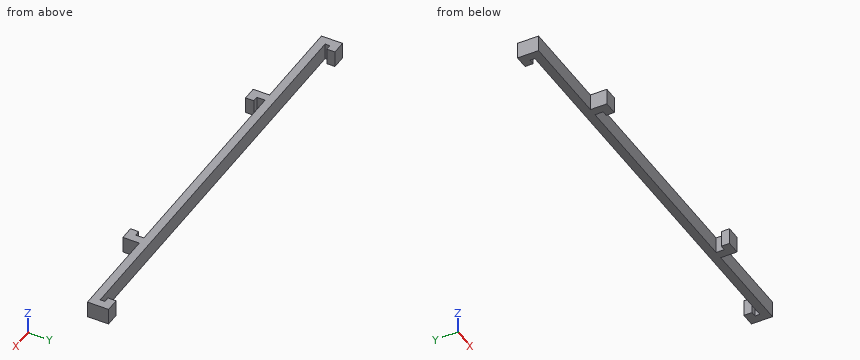
from build123d import *

# Parameters (mm, degrees)
F1_DEPTH = 6


with BuildPart() as f1:
    # F0 (on Top) → F1 (new body)
    with BuildSketch(Plane.XY):
        Polygon((-72.304564, 6.418628), (-72.304564, 9.418628), (-77.304564, 9.418628), (-77.304564, 1.718628), (-43.054564, 1.718628), (-43.054564, -4.281372), (-38.054564, -4.281372), (-38.054564, -1.281372), (-40.054564, -1.281372), (-40.054564, 1.718628), (39.945436, 1.718628), (39.945436, -1.281372), (37.945436, -1.281372), (37.945436, -4.281372), (42.945436, -4.281372), (42.945436, 1.718628), (77.195436, 1.718628), (77.195436, 9.418628), (72.195436, 9.418628), (72.195436, 6.418628), (74.195436, 6.418628), (74.195436, 4.718628), (-74.304564, 4.718628), (-74.304564, 6.418628), align=None)
    extrude(amount=F1_DEPTH)


solid = f1.part
Verification items for the finished model (mm, model axes). Give positions to 0.01 mm unless a question says otherwise; leave off trailing zeros. Loops run counter-clockwise (first coordinate to the right, second up) from the corner with the lowest first, then second, coordinate; pieces in that order, holes last. Notation, with made-up numbers: (28.25, 42.5) - (38.25, 42.5) arc R9 ccw to (38.25, 46.5) - close; hole circle Ø11 at (33.5, 80.5). An arc over 180 degrees is marked (long way). Write item = value, one per line. Start each with the question number.
Q1. Cross-section at C-C, the plane x = 52. Enter the section's corners in (y, z), and give its area (3 significant figures).
Q2. Cross-section at B-B, the plane z = 4.8. Enter the section's corners in (x, y), and give its area (3 significant figures).
Q3. Cross-section at A-A, the plane y = 0. Enter the section's corners in (x, z).
Q4. Depth check by flat-ended pin: P1, Ø2.5, axis at y = -3, z = 1.5, coming from the +X side; P2, Ø3, axis at y = -2.5, z = 2, coming from the -X side; P3, Ø2, axis at x = -38.5, z = 2.5, coming from the +Y side. Enter the tip coordinate at first touch or a pass-through.
Q5. Thickness scan on line 1 (X direction, y = 8.5, z = 5.3); line 2 (X direction, y = -1.25, z = 2.85); line 3 (Y direction, x = 32, z = 5.5). Record the ranges inside material, lowest first.
Answer key:
q1.outline = (1.72, 0) - (4.72, 0) - (4.72, 6) - (1.72, 6) - close
q1.area = 18.0 mm^2
q2.outline = (-77.3, 1.72) - (-43.05, 1.72) - (-43.05, -4.28) - (-38.05, -4.28) - (-38.05, -1.28) - (-40.05, -1.28) - (-40.05, 1.72) - (39.95, 1.72) - (39.95, -1.28) - (37.95, -1.28) - (37.95, -4.28) - (42.95, -4.28) - (42.95, 1.72) - (77.2, 1.72) - (77.2, 9.42) - (72.2, 9.42) - (72.2, 6.42) - (74.2, 6.42) - (74.2, 4.72) - (-74.3, 4.72) - (-74.3, 6.42) - (-72.3, 6.42) - (-72.3, 9.42) - (-77.3, 9.42) - close
q2.area = 552 mm^2
q3.outline = (-43.05, 0) - (-40.05, 0) - (-40.05, 6) - (-43.05, 6) - close; (39.95, 0) - (42.95, 0) - (42.95, 6) - (39.95, 6) - close
q4.P1 = 42.95
q4.P2 = -43.05
q4.P3 = 4.72
q5.line_1 = -77.3 to -72.3, 72.2 to 77.2
q5.line_2 = -43.05 to -40.05, 39.95 to 42.95
q5.line_3 = 1.72 to 4.72
